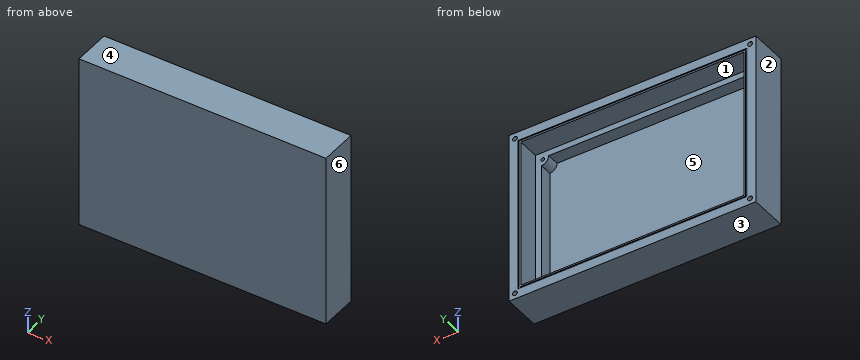
Autodesk Inventor part; units mm, degrees
ref_plane "YZ Plane" through (0, 0, 0) normal (1, 0, 0) x (0, 1, 0)
ref_plane "XZ Plane" through (0, 0, 0) normal (0, 1, 0) x (-1, 0, 0)
ref_plane "XY Plane" through (0, 0, 0) normal (0, 0, 1) x (1, 0, 0)
sketch "Esboço9" plane through (0, 0, 0) normal (0, 1, 0) x (-1, 0, 0)
  line L0 (123.7607, -142.906) -> (-28.2393, -142.906)
  line L1 (-28.2393, -142.906) -> (-28.2393, -40.906)
  line L2 (-28.2393, -40.906) -> (123.7607, -40.906)
  line L3 (123.7607, -40.906) -> (123.7607, -142.906)
  point P0 (0, 0)
  dimension "d42" = 152
  dimension "d43" = 102
extrude "Extrusão7" add sketch "Esboço9" along normal blind 10.6
shell "Casca2" thickness 2 removed faces 1 at (-22.4273, 10.6, -74.906)
sketch "Esboço10" plane through (0, 10.6, 0) normal (0, 1, 0) x (1, 0, 0)
  line L0 (-123.7607, 142.906) -> (-123.7607, 40.906)
  line L1 (-123.7607, 40.906) -> (28.2393, 40.906)
  line L2 (28.2393, 142.906) -> (-123.7607, 142.906)
  line L3 (28.2393, 40.906) -> (28.2393, 142.906)
  line L4 (-123.7607, 40.906) -> (-131.7607, 40.906)
  line L5 (-131.7607, 40.906) -> (-131.7607, 142.906)
  line L6 (-131.7607, 142.906) -> (-123.7607, 142.906)
  line L7 (-123.7607, 142.906) -> (-123.7607, 40.906)
  line L8 (-131.7607, 142.906) -> (28.2393, 142.906)
  line L9 (28.2393, 142.906) -> (28.2393, 150.906)
  line L10 (28.2393, 150.906) -> (-131.7607, 150.906)
  line L11 (-131.7607, 150.906) -> (-131.7607, 142.906)
  line L12 (28.2393, 40.906) -> (36.2393, 40.906)
  line L13 (36.2393, 40.906) -> (36.2393, 150.906)
  line L14 (36.2393, 150.906) -> (28.2393, 150.906)
  line L15 (28.2393, 150.906) -> (28.2393, 40.906)
  line L16 (-131.7607, 40.906) -> (36.2393, 40.906)
  line L17 (36.2393, 40.906) -> (36.2393, 32.906)
  line L18 (36.2393, 32.906) -> (-131.7607, 32.906)
  line L19 (-131.7607, 32.906) -> (-131.7607, 40.906)
  point P0 (0, 0)
  dimension "d47" = 8
  dimension "d48" = 8
  dimension "d49" = 8
  dimension "d50" = 8
extrude "Extrusão8" add sketch "Esboço10" along normal blind 15 and the other way blind 10.6 contours L6 L11 L10 L9 L2 | L0 L4 L5 L6 | L1 L12 L17 L18 L19 L4 | L9 L14 L13 L12 L3
sketch "Esboço11" plane through (0, 10.6, 0) normal (0, 1, 0) x (1, 0, 0)
  line L0 (-121.7607, 42.906) -> (-121.7607, 140.906)
  line L1 (26.2393, 42.906) -> (-121.7607, 42.906)
  line L2 (-121.7607, 140.906) -> (26.2393, 140.906)
  line L3 (26.2393, 140.906) -> (26.2393, 42.906)
  line L4 (-121.7607, 42.906) -> (-119.7607, 42.906)
  line L5 (-119.7607, 42.906) -> (-119.7607, 140.906)
  line L6 (-119.7607, 140.906) -> (-121.7607, 140.906)
  line L7 (-121.7607, 140.906) -> (-121.7607, 42.906)
  line L8 (26.2393, 140.906) -> (-121.7607, 140.906)
  line L9 (-121.7607, 140.906) -> (-121.7607, 138.906)
  line L10 (-121.7607, 138.906) -> (26.2393, 138.906)
  line L11 (26.2393, 138.906) -> (26.2393, 140.906)
  line L12 (-121.7607, 42.906) -> (26.2393, 42.906)
  line L13 (26.2393, 42.906) -> (26.2393, 44.906)
  line L14 (26.2393, 44.906) -> (-121.7607, 44.906)
  line L15 (-121.7607, 44.906) -> (-121.7607, 42.906)
  line L16 (26.2393, 42.906) -> (24.2393, 42.906)
  line L17 (24.2393, 42.906) -> (24.2393, 140.906)
  line L18 (24.2393, 140.906) -> (26.2393, 140.906)
  line L19 (26.2393, 140.906) -> (26.2393, 42.906)
  point P0 (0, 0)
  point P1 (-119.7607, 138.906)
  point P2 (24.2393, 138.906)
  point P3 (24.2393, 44.906)
  point P4 (-119.7607, 44.906)
  dimension "d55" = 2
  dimension "d56" = 2
  dimension "d57" = 2
  dimension "d58" = 2
extrude "Extrusão9" add sketch "Esboço11" against normal blind 8.6 contours L0 L14 L5 L1 | L0 L10 L5 L14 | L5 L14 L17 L1 | L0 L2 L5 L10 | L17 L14 L3 L1 | L5 L2 L17 L10 | L17 L10 L3 L14 | L17 L2 L3 L10
sketch "Esboço12" plane through (0, 10.6, 0) normal (0, 1, 0) x (1, 0, 0)
  line L0 (24.2393, 138.906) -> (24.2393, 44.906)
  line L1 (24.2393, 44.906) -> (-119.7607, 44.906)
  line L2 (-119.7607, 138.906) -> (24.2393, 138.906)
  line L3 (-119.7607, 44.906) -> (-119.7607, 138.906)
  arc A0 (19.2393, 138.906) -> (24.2393, 133.906) centre (24.2393, 138.906) ccw
  arc A1 (24.2393, 49.906) -> (19.2393, 44.906) centre (24.2393, 44.906) ccw
  arc A2 (-114.7607, 44.906) -> (-119.7607, 49.906) centre (-119.7607, 44.906) ccw
  arc A3 (-119.7607, 133.906) -> (-114.7607, 138.906) centre (-119.7607, 138.906) ccw
  point P0 (0, 0)
  dimension "d61" = 5
  dimension "d62" = 5
  dimension "d63" = 5
  dimension "d64" = 5
extrude "Extrusão10" add sketch "Esboço12" against normal blind 8.6 contours L0 A0 L2 | L0 L1 A1 | A3 L3 L2 | L1 L3 A2
sketch "Esboço13" plane through (0, 10.6, 0) normal (0, 1, 0) x (1, 0, 0)
  line L0 (28.2393, 40.906) -> (28.2393, 142.906)
  line L1 (-123.7607, 40.906) -> (28.2393, 40.906)
  point P0 (0, 0)
  point P1 (23.2393, 45.906)
  dimension "d67" = 5
  dimension "d68" = 5
hole "Furo2" at (23.2393, 10.6, -45.906) direction (0, -1, 0) diameter 2.459 depth 5 tip angle 118
sketch "Esboço14" plane through (0, 10.6, 0) normal (0, 1, 0) x (1, 0, 0)
  line L0 (28.2393, 40.906) -> (28.2393, 142.906)
  line L1 (28.2393, 142.906) -> (-123.7607, 142.906)
  point P0 (0, 0)
  point P1 (23.2393, 137.906)
  dimension "d76" = 5
  dimension "d77" = 5
hole "Furo3" at (23.2393, 10.6, -137.906) direction (0, -1, 0) diameter 2.459 depth 5 tip angle 118
sketch "Esboço15" plane through (0, 10.6, 0) normal (0, 1, 0) x (1, 0, 0)
  line L0 (28.2393, 142.906) -> (-123.7607, 142.906)
  line L1 (-123.7607, 142.906) -> (-123.7607, 40.906)
  point P0 (0, 0)
  point P1 (-118.7607, 137.906)
  dimension "d85" = 5
  dimension "d86" = 5
hole "Furo4" at (-118.7607, 10.6, -137.906) direction (0, -1, 0) diameter 2.459 depth 5 tip angle 118
sketch "Esboço16" plane through (0, 10.6, 0) normal (0, 1, 0) x (1, 0, 0)
  line L0 (-123.7607, 142.906) -> (-123.7607, 40.906)
  line L1 (-123.7607, 40.906) -> (28.2393, 40.906)
  point P0 (0, 0)
  point P1 (-118.7607, 45.906)
  dimension "d94" = 5
  dimension "d95" = 5
hole "Furo5" at (-118.7607, 10.6, -45.906) direction (0, -1, 0) diameter 2.459 depth 5 tip angle 118
sketch "Esboço18" plane through (0, 25.6, 0) normal (0, 1, 0) x (1, 0, 0)
  point P0 (0, 0)
sketch "Esboço19" plane through (0, 25.6, 0) normal (0, 1, 0) x (1, 0, 0)
  point P0 (0, 0)
sketch "Esboço20" plane through (0, 25.6, 0) normal (0, 1, 0) x (1, 0, 0)
  line L0 (-131.7607, 32.906) -> (36.2393, 32.906)
  line L1 (-131.7607, 150.906) -> (-131.7607, 32.906)
  point P0 (0, 0)
  point P1 (-127.7607, 36.906)
  dimension "d104" = 4
  dimension "d105" = 4
hole "Furo6" at (-127.7607, 25.6, -36.906) direction (0, -1, 0) diameter 3.242 depth 15 tip angle 118
sketch "Esboço21" plane through (0, 25.6, 0) normal (0, 1, 0) x (1, 0, 0)
  line L0 (28.2393, 142.906) -> (28.2393, 40.906)
  line L1 (-124.3607, 143.906) -> (28.8393, 143.906)
  line L2 (29.2393, 143.506) -> (29.2393, 40.306)
  line L3 (28.8393, 39.906) -> (-124.3607, 39.906)
  line L4 (-124.7607, 40.306) -> (-124.7607, 143.506)
  line L5 (-125.2607, 39.006) -> (29.7393, 39.006)
  line L6 (30.1393, 39.406) -> (30.1393, 144.406)
  line L7 (29.7393, 144.806) -> (-125.2607, 144.806)
  line L8 (-125.6607, 144.406) -> (-125.6607, 39.406)
  arc A0 (-125.6607, 39.406) -> (-125.2607, 39.006) centre (-125.2607, 39.406) ccw
  arc A1 (-124.7607, 40.306) -> (-124.3607, 39.906) centre (-124.3607, 40.306) ccw
  arc A2 (-124.3607, 143.906) -> (-124.7607, 143.506) centre (-124.3607, 143.506) ccw
  arc A3 (-125.2607, 144.806) -> (-125.6607, 144.406) centre (-125.2607, 144.406) ccw
  arc A4 (28.8393, 39.906) -> (29.2393, 40.306) centre (28.8393, 40.306) ccw
  arc A5 (29.7393, 39.006) -> (30.1393, 39.406) centre (29.7393, 39.406) ccw
  arc A6 (29.2393, 143.506) -> (28.8393, 143.906) centre (28.8393, 143.506) ccw
  arc A7 (30.1393, 144.406) -> (29.7393, 144.806) centre (29.7393, 144.406) ccw
  point P0 (0, 0)
  point P1 (-123.7607, 40.906)
  dimension "d117" = 0.9
  dimension "d118" = 0.4
extrude "Extrusão11" cut sketch "Esboço21" against normal blind 0.6
sketch "Esboço22" plane through (0, 25.6, 0) normal (0, 1, 0) x (1, 0, 0)
  line L0 (-131.7607, 150.906) -> (-131.7607, 32.906)
  line L1 (36.2393, 150.906) -> (-131.7607, 150.906)
  line L2 (36.2393, 32.906) -> (36.2393, 150.906)
  line L3 (-131.7607, 32.906) -> (36.2393, 32.906)
  point P0 (0, 0)
  point P1 (-127.7607, 146.906)
  point P2 (32.2393, 146.906)
  point P3 (32.2393, 36.906)
  dimension "d121" = 4
  dimension "d122" = 4
  dimension "d123" = 4
  dimension "d124" = 4
  dimension "d125" = 4
  dimension "d126" = 4
hole "Furo7" at (-127.7607, 25.6, -146.906) at (32.2393, 25.6, -146.906) at (32.2393, 25.6, -36.906) direction (0, -1, 0) diameter 3.242 depth 15 tip angle 118
properties part number "peça pi2"
The model under review builds one solid part; all positions refer to its coordinate system, in mm. Face numbers are marked on the shaded views. A direction names the side the tool comes from. Coordinates: 2 decimals unless noted, no trailing zeros. Order: outer loops, then holes, each group sorted by start corner. A loop starts at its lowest first (then second) coordinate and runs counter-clockwise, first axis right, second up. Notation, with made-up numbers: (-6.75, -20) -> (-0.75, -20) arc R25 cw to (-0.75, 4) -> close; hole circle Ø10 at (-15, -9). An arc over 180 degrees is marked (long way). Answer in a Markdown table with one row per item. Add a question column.
Item 1: Machinability: for the marked faces 5 and 6, which of the approach directions +Z, -Z, +X, -X, +Y, -Y give a long, thin tool a straight path to every point of the face, cutting with its end or side? Answer none if there is none.
Item 2: We need section B-B on x = -86.5. Write out the cut boundary in (y, z), plus the area to 3 significant figures.
Item 3: To check wall thickness, follow probe 1 along Z at (x, y) = (-88.5, 8); probe 2 along X at (y, z) = (7.25, -124); probe 3 along X at (y, z) = (14.5, -142.5). State the ranges of each line that lie inside material, in increasing order.
Item 4: We need section D-D on y = 7.5. Write out the cut boundary in (x, z).
Item 5: We need section C-C on y = 23. Write out the cut boundary in (x, z) (3 decimals).
Item 6: Mouldability with a two-part tool opening along Z and no side actions: class the marked faces 1, 2, 3 and 4 as +Z half, -Z half, draft (parallel to the pull), parting line (faces both ways), or undercut.
Item 7: Clearance check with a flat-ended pin moving along its axis: pin 1 (3 mm diameter, centred on x = -106.5, z = -63, fed in from +Y). State where the tip first meets the part, or that it passes through.
Item 8: We need section A-A on z = -79. Write out the cut boundary in (x, y), plus the area to 3 significant figures.
Final values:
| question | item | result |
|---|---|---|
| 1 | face 5 | +Y |
| 1 | face 6 | +Z, -Z, +X, +Y, -Y |
| 2 | outline | (0, -150.91) -> (25.6, -150.91) -> (25.6, -144.81) -> (25, -144.81) -> (25, -143.91) -> (25.6, -143.91) -> (25.6, -142.91) -> (10.6, -142.91) -> (10.6, -138.91) -> (2, -138.91) -> (2, -44.91) -> (10.6, -44.91) -> (10.6, -40.91) -> (25.6, -40.91) -> (25.6, -39.91) -> (25, -39.91) -> (25, -39.01) -> (25.6, -39.01) -> (25.6, -32.91) -> (0, -32.91) -> close |
| 2 | area | 681 mm2 |
| 3 | probe 1 | z = -150.91 to -138.91, -44.91 to -32.91 |
| 3 | probe 2 | x = -131.76 to -119.76, 24.24 to 36.24 |
| 3 | probe 3 | x = -131.76 to -123.76, 28.24 to 36.24 |
| 4 | outline | (-131.76, -150.91) -> (36.24, -150.91) -> (36.24, -32.91) -> (-131.76, -32.91) -> close; hole circle Ø2.46 at (-118.76, -137.91); hole circle Ø2.46 at (-118.76, -45.91); hole (-119.76, -133.91) arc R5 cw to (-114.76, -138.91) -> (19.24, -138.91) arc R5 cw to (24.24, -133.91) -> (24.24, -49.91) arc R5 cw to (19.24, -44.91) -> (-114.76, -44.91) arc R5 cw to (-119.76, -49.91) -> close; hole circle Ø2.46 at (23.24, -137.91); hole circle Ø2.46 at (23.24, -45.91) |
| 5 | outline | (-131.761, -150.906) -> (36.239, -150.906) -> (36.239, -32.906) -> (-131.761, -32.906) -> close; hole circle Ø3.242 at (-127.761, -146.906); hole circle Ø3.242 at (-127.761, -36.906); hole (-123.761, -142.906) -> (28.239, -142.906) -> (28.239, -40.906) -> (-123.761, -40.906) -> close; hole circle Ø3.242 at (32.239, -146.906); hole circle Ø3.242 at (32.239, -36.906) |
| 6 | face 1 | undercut |
| 6 | face 2 | draft |
| 6 | face 3 | -Z half |
| 6 | face 4 | +Z half |
| 7 | pin 1 | stops at y = 2 |
| 8 | outline | (-131.76, 0) -> (36.24, 0) -> (36.24, 25.6) -> (30.14, 25.6) -> (30.14, 25) -> (29.24, 25) -> (29.24, 25.6) -> (28.24, 25.6) -> (28.24, 10.6) -> (24.24, 10.6) -> (24.24, 2) -> (-119.76, 2) -> (-119.76, 10.6) -> (-123.76, 10.6) -> (-123.76, 25.6) -> (-124.76, 25.6) -> (-124.76, 25) -> (-125.66, 25) -> (-125.66, 25.6) -> (-131.76, 25.6) -> close |
| 8 | area | 781 mm2 |
